from build123d import *

# Parameters (mm, degrees)
F1_DEPTH = 1524
F3_DEPTH = 101.6


with BuildPart() as f1:
    # F0 (on Right) → F1 (new body)
    with BuildSketch(Plane.YZ):
        with BuildLine():
            Line((-627.0625, 0), (0, 0))
            Line((0, 0), (0, 31.75))
            Line((0, 31.75), (-627.0625, 31.75))
            ThreePointArc((-627.0625, 31.75), (-642.9375, 15.875), (-627.0625, 0))
        make_face()
    extrude(amount=F1_DEPTH)

    # F2 (on face) → F3 (join)
    with BuildSketch(Plane.XY.offset(31.75)):
        Polygon((19.9898, -627.0625), (19.9898, -19.9898), (1524, -19.9898), (1524, 0), (0, 0), (0, -627.0625), align=None)
    extrude(amount=F3_DEPTH)


solid = f1.part
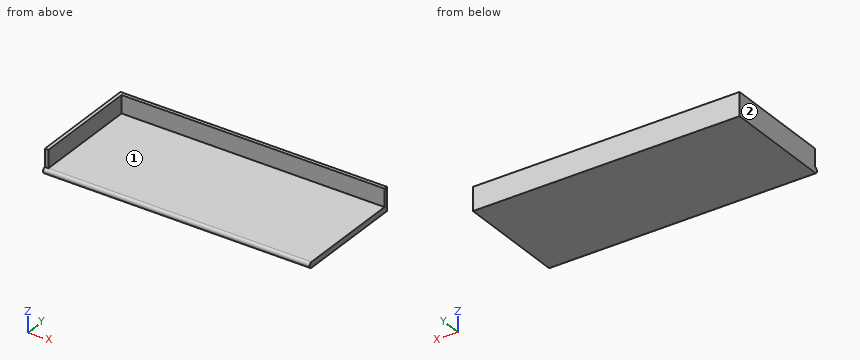
Model file for the job. Use its own axes, mm. Face numbers are marked on the shaded views. A direction names the side the tool comes from. Round coordinates to 2 decimals unless told otherwise and drop trailing zeros. Order: outer loops, then holes, each group sorted by start corner. A loop starts at its lowest first (then second) coordinate and runs counter-clockwise, first axis right, second up.
(1) 3-axis set-ups, long thin cutter, end or side, ignore diameter. For the marked faces 1 and 2: which of +Z, -Z, +X, -X, +Y, -Y reach the whole face in a straight line?
(2) Pin check, flat tips, straight feed: pin 1 (1.5 mm diameter, centred on y = -73.5, z = 113, fed in from +X); pin 2 (3 mm diameter, centred on x = 476.5, z = 94, fed in from -Y); pin 3 (10 mm diameter, centred on x = 751.5, y = -455.5, fed in from +Z). Stop position of each tip, or through.
(3) Band-saw the part on B-B (z = 94). List the corners of the cut face in (x, y), then the cut area to 3 significant figures.
(4) Drill centre lines: line 1 (Z direction, x = 1164, y = -600); line 2 (Y direction, x = 1076.5, z = 42); line 3 (X direction, y = -167.5, z = 76). Where is each one in solid material? Low to high.
Verdict:
1. face 1: +Z, +X, -Y
1. face 2: +Z, -Z, -X, +Y, -Y
2. pin 1: stops at x = 19.99
2. pin 2: stops at y = -19.99
2. pin 3: stops at z = 31.75
3. outline: (0, -627.06) - (19.99, -627.06) - (19.99, -19.99) - (1524, -19.99) - (1524, 0) - (0, 0) - close
3. area: 42,600 mm2
4. line 1: z = 0 to 31.75
4. line 2: y = -19.99 to 0
4. line 3: x = 0 to 19.99
